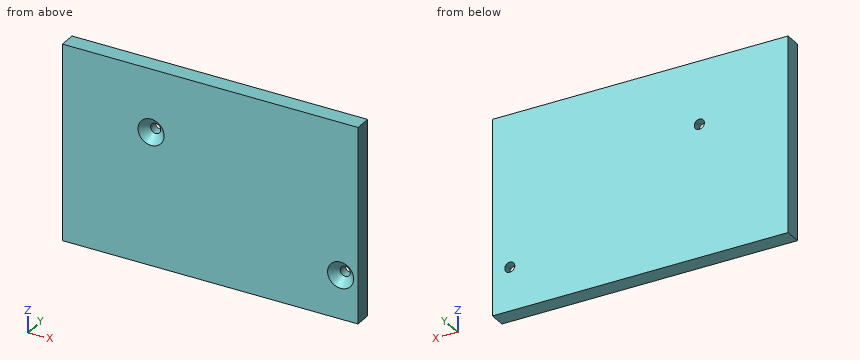
```python
from build123d import *

# Parameters (mm, degrees)
SKETCH1_W                                         = 85
SKETCH1_H                                         = 56
BOSS_EXTRUDE1_DEPTH                               = 4.7625
CSK_FOR_M2_5_FLAT_HEAD_MACHINE_SCREW1_D           = 2.9
CSK_FOR_M2_5_FLAT_HEAD_MACHINE_SCREW1_CSINK_D     = 7.5
CSK_FOR_M2_5_FLAT_HEAD_MACHINE_SCREW1_CSINK_ANGLE = 90


with BuildPart() as part:
    # Sketch1 → Boss-Extrude1 (new body)
    with BuildSketch(Plane(origin=(0, 0, 0), x_dir=(1, 0, 0), z_dir=(0, 1, 0))):
        Rectangle(SKETCH1_W, SKETCH1_H)
    extrude(amount=BOSS_EXTRUDE1_DEPTH)

    # CSK for M2.5 Flat Head Machine Screw1 (through all)
    with Locations(Plane(origin=(-17, 0, 10), x_dir=(0, 0, -1), z_dir=(0, -1, 0))):
        with Locations((0, 0), (25.5, 54.5)):
            CounterSinkHole(CSK_FOR_M2_5_FLAT_HEAD_MACHINE_SCREW1_D / 2, CSK_FOR_M2_5_FLAT_HEAD_MACHINE_SCREW1_CSINK_D / 2, counter_sink_angle=CSK_FOR_M2_5_FLAT_HEAD_MACHINE_SCREW1_CSINK_ANGLE)


solid = part.part
```
Can you work these out from the model? Positions are in its coordinate system, mm. Round coordinates to 2 decimals unless told otherwise and drop trailing zeros. Loops run counter-clockwise (first coordinate to the right, second up) from the corner with the lowest first, then second, coordinate; pieces in that order, holes last. Notation, with made-up numbers: M 81,-20 L 86,-20 A20 ccw 86,-8 Z; hole C 33,6 d2. An arc over 180 degrees is marked long. Answer as a JSON object with one key per item and string values. Group by question number.
Q1. Imagine slicing it at B-B, the plane x = -17. Please give me the cut outline in (y, z), then the cut area to 3 significant figures.
Q2. Will these pins go through, and if not, where does the flat tip stop? pin 1 (2.5 mm diameter, centred on x = 37.5, z = -15.5, fed in from -Y); pin 2 (3.5 mm diameter, centred on x = -17, z = 10, fed in from -Y).
Q3. Imagine slicing it at A-A, the plane z = 10. Please give me the cut outline in (x, y), then the cut area to 3 significant figures.
Q4. Please list where these lines run through material, in increasing order: L1, parallel to X at y = 4.1, z = 10; L2, parallel to X at y = 3.3, z = -15.5; L3, parallel to Z at x = 37.5, y = 3.
Findings:
{
 "1": {"outline": "M 0,-28 L 4.76,-28 L 4.76,8.55 L 2.3,8.55 L 0,6.25 Z; M 0,13.75 L 2.3,11.45 L 4.76,11.45 L 4.76,28 L 0,28 Z", "area": "248 mm2"},
 "2": {"pin 1": "passes through", "pin 2": "stops at y = 2"},
 "3": {"outline": "M -42.5,0 L -20.75,0 L -18.45,2.3 L -18.45,4.76 L -42.5,4.76 Z; M -15.55,2.3 L -13.25,0 L 42.5,0 L 42.5,4.76 L -15.55,4.76 Z", "area": "386 mm2"},
 "4": {"L1": "x = -42.5 to -18.45, -15.55 to 42.5", "L2": "x = -42.5 to 36.05, 38.95 to 42.5", "L3": "z = -28 to -16.95, -14.05 to 28"}
}
